Could you check a few things on this model? Use its own coordinates, in mm. A direction names the side the tool comes from. Give positions to 0.01 mm unless a question says otherwise; leave off trailing zeros. Order: outer loops, then holes, each group sorted by start corner. A loop starts at its lowest first (then second) coordinate and runs counter-clockwise, first axis right, second up.
from build123d import *

# Parameters (mm, degrees)
EXTRUDE_1_DEPTH = 1
SKETCH_2_W      = 12.935520023
SKETCH_2_H      = 10.454735361
EXTRUDE_2_DEPTH = 6


with BuildPart() as part:
    # Эскиз1 → Бобышка-Вытянуть1 (new body)
    with BuildSketch(Plane.XY):
        with BuildLine():
            Line((0, 0), (19.35, 0))
            ThreePointArc((19.35, 0), (20.8, 1.45), (22.25, 0))
            Line((22.25, 0), (33, 0))
            Line((33, 0), (33, 28))
            Line((33, 28), (22.25, 28))
            ThreePointArc((22.25, 28), (20.8, 26.55), (19.35, 28))
            Line((19.35, 28), (0, 28))
            Line((0, 28), (0, 15.45))
            ThreePointArc((0, 15.45), (1.45, 14), (0, 12.55))
            Line((0, 12.55), (0, 0))
        make_face()
    extrude(amount=EXTRUDE_1_DEPTH)

    # Эскиз2 → Бобышка-Вытянуть2 (add)
    with BuildSketch(Plane.XY.offset(1)):
        with Locations((10.395518043, 21.660261576)):
            Rectangle(SKETCH_2_W, SKETCH_2_H)
    extrude(amount=EXTRUDE_2_DEPTH)


solid = part.part
Item 1: Imagine slicing it at C-C on z = 3.75. List the corners of the cut face in (x, y) for me.
Findings:
outline: (3.93, 16.43) - (16.86, 16.43) - (16.86, 26.89) - (3.93, 26.89) - close
Item 2: Imagine slicing it at D-D on x = 25.5. List the corners of the cut face in (y, z) for me.
Findings:
outline: (0, 0) - (28, 0) - (28, 1) - (0, 1) - close
Item 3: Imagine slicing it at B-B on x = 8.5. List the corners of the cut face in (y, z) for me.
Findings:
outline: (0, 0) - (28, 0) - (28, 1) - (26.89, 1) - (26.89, 7) - (16.43, 7) - (16.43, 1) - (0, 1) - close
Item 4: Imagine slicing it at A-A on y = 21.5. List the corners of the cut face in (x, z) for me, then the cut area to 3 significant figures.
Findings:
outline: (0, 0) - (33, 0) - (33, 1) - (16.86, 1) - (16.86, 7) - (3.93, 7) - (3.93, 1) - (0, 1) - close
area: 111 mm2
Item 5: For faces 1 (the flat face through (3.928, 22, 4)), 2 (the flat face through (9.8, 28, 0.5)), 3 (the flat face through (16.863, 22, 4)), 4 (the flat face through (10, 16.433, 4)), which set-ups out of +Z, -Z, +X, -X, +Y, -Y let a thin tool reach every point of the face, with its end or its side?
Findings:
face 1: +Z, -X, +Y, -Y
face 2: +Z, -Z, +X, -X, +Y
face 3: +Z, +X, +Y, -Y
face 4: +Z, +X, -X, -Y
Item 6: Please list where these lines run through material, in increasing order: line 1 along Z through (x, y) = (17.5, 8); line 2 along X through (y, z) = (18.5, 1.5); line 3 along Y through (x, z) = (15, 3.75).
Findings:
line 1: z = 0 to 1
line 2: x = 3.93 to 16.86
line 3: y = 16.43 to 26.89
Item 7: For pin 1 (3 mm diameter, centred on y = 10, z = 1.5, fed in from -X); pin 2 (1 mm diameter, centred on y = 16, z = 5.5, fed in from -X); pin 3 (2 mm diameter, centred on x = 10.5, z = 5.5, fed in from +Y); pin 4 (12 mm diameter, centred on x = 28, y = 24.5, fed in from +Z), each with a flat end and sliding along its axis, tell me the tip position at first contact or that it passes through.
Findings:
pin 1: stops at x = 0
pin 2: stops at x = 3.93
pin 3: stops at y = 26.89
pin 4: stops at z = 1
Item 8: We'd pull the mould along Y, two halves only. Please class faces 5 (the flat face through (10, 26.888, 4)), 6 (the flat face through (27.5, 0, 0.5)), 7 (the flat face through (0, 21.8, 0.5)), 8 (the cylindrical face through (1.45, 14.03, 0.49)): +Y half, -Y half, draft (parallel to the pull), parting line (faces both ways), or undercut.
Findings:
face 5: +Y half
face 6: -Y half
face 7: draft
face 8: undercut
